The listing builds one solid part. Answer for the finished solid, in the listing's coordinates (mm). A direction names the side the tool comes from. Give positions to 0.01 mm unless a question says otherwise; leave off trailing zeros. Loops run counter-clockwise (first coordinate to the right, second up) from the corner with the lowest first, then second, coordinate; pieces in that order, holes last.
Item 1: Consider line 1 along Y through (x, z) = (25, 1.25) (3 decimals); line 2 along X through (y, z) = (5.75, 0.95); line 3 along X through (y, z) = (10.5, 3.75). Determine where each line is inside the solid, lowest interval first.
Item 2: Section A-A, the plane x = 22 is taken. Give the vertices of the cut face in (y, z) (3 decimals), and give its area (3 significant figures).
Item 3: A tool of negligible diameter and unlimited length cuts with its end or side. For faces 1 (the face through (25.15, 6, 3)), 2 (the face through (44, 3.425, 3)), 3 (the face through (3, 3.425, 3)), from which of +Z, -Z, +X, -X, +Y, -Y can it reach the whole face along a straight path? Write none if from no direction.
Item 4: The mould has two halves that part along X. Classify faces 4 (the face through (23, 9, 5.15)), 5 (the face through (23, 3.425, 3)), 6 (the face through (23, 8.575, 3)), 7 (the face through (5.15, 10, 3)): pulls with the +X half, pulls with the -X half, needs draft (parallel to the pull), parting line crosses it, or undercut.
Item 5: Section C-C, the plane y = 9 is taken. Give the vertices of the cut face in (x, z).
Item 6: Section B-B, the plane z = 4.15 is taken. Give the vertices of the cut face in (x, y) (3 decimals).
Item 7: Each of these flat-tipped pins is pushed along its axis until it touches: pin 1 Ø1.5 at (x, z) = (43.5, 2) entering from -Y (3 decimals); pin 2 Ø1 at (y, z) = (10.5, 1.5) entering from +X; pin 3 Ø2.5 at (y, z) = (2, 2.5) entering from -X. Where does it stop, or does it pass through?
from build123d import *

# Parameters (mm, degrees)
BOSS_EXTRUDE1_DEPTH = 5.15
SKETCH3_W           = 5.15
SKETCH3_H           = 5.15
CUT_EXTRUDE1_DEPTH  = 6.15


with BuildPart() as part:
    # Sketch2 → Boss-Extrude1 (new body)
    with BuildSketch(Plane.XY):
        Polygon((0, 3.425), (0, 8.575), (5.15, 8.575), (5.15, 12), (41.15, 12), (41.15, 8.575), (46.3, 8.575), (46.3, 3.425), (41.15, 3.425), (41.15, 0), (5.15, 0), (5.15, 3.425), align=None)
    extrude(amount=BOSS_EXTRUDE1_DEPTH)

    # Sketch3 → Cut-Extrude1 (cut, through all)
    with BuildSketch(Plane.XY.offset(5.15)):
        with Locations((22.575, 6)):
            Rectangle(SKETCH3_W, SKETCH3_H)
    extrude(amount=-CUT_EXTRUDE1_DEPTH, mode=Mode.SUBTRACT)


solid = part.part
Worked answers:
1. line 1: y = 0 to 3.425, 8.575 to 12
1. line 2: x = 0 to 20, 25.15 to 46.3
1. line 3: x = 5.15 to 41.15
2. outline: (0, 0) - (3.425, 0) - (3.425, 5.15) - (0, 5.15) - close; (8.575, 0) - (12, 0) - (12, 5.15) - (8.575, 5.15) - close
2. area: 35.3 mm2
3. face 1: +Z, -Z
3. face 2: +Z, -Z, +X, -Y
3. face 3: +Z, -Z, -X, -Y
4. face 4: needs draft
4. face 5: undercut
4. face 6: undercut
4. face 7: pulls with the -X half
5. outline: (5.15, 0) - (41.15, 0) - (41.15, 5.15) - (5.15, 5.15) - close
6. outline: (0, 3.425) - (5.15, 3.425) - (5.15, 0) - (41.15, 0) - (41.15, 3.425) - (46.3, 3.425) - (46.3, 8.575) - (41.15, 8.575) - (41.15, 12) - (5.15, 12) - (5.15, 8.575) - (0, 8.575) - close; hole (20, 3.425) - (25.15, 3.425) - (25.15, 8.575) - (20, 8.575) - close
7. pin 1: stops at y = 3.425
7. pin 2: stops at x = 41.15
7. pin 3: stops at x = 5.15
